Read the model definition and answer for the solid it produces. Units are mm, in the model's axes. Coordinates: 2 decimals unless noted, no trailing zeros. Write each loop counter-clockwise with the first axis right and the second up, starting at its lowest first coordinate (ties: lowest second). Pieces come first, ordered by that corner, then holes.
Item 1: Section B-B (z = 30) is taken. Give the vertices of the cut face in (x, y), then the cut area to 3 significant figures.
Item 2: Determine the mould class of faces 1 (the face through (1, 322.58, 9)), 2 (the face through (-25.97, 159.03, -33.86)), 3 (the face through (14, 159, 0)) for opening direction X: released by +X, released by -X, zero draft, split by the parting line, or undercut.
Item 3: Straight lines are drawn through the part: probe 1 along Z at (x, y) = (12, 136); probe 2 along Z at (x, y) = (-5, 158.5); probe 3 along X at (y, z) = (225, -16.5). For each, find the intervals that lie inside material, in ascending order.
Item 4: Section C-C (x = -25) is taken. Give the vertices of the cut face in (y, z).
Item 5: Each of these flat-tipped pins is pushed along its axis until it touches: P1, Ø12.5, axis at y = 134, z = 13.5, coming from the -X side; P2, Ø5, axis at y = 138.5, z = 31, coming from the +X side; P3, Ø17.5, axis at x = -13, y = 170, coming from the +Z side. Where does it stop, or does it pass through?
from build123d import *

# Parameters (mm, degrees)
SKETCH1_R           = 42.672
BOSS_EXTRUDE1_DEPTH = 322.58


with BuildPart() as part:
    # Sketch1 → Boss-Extrude1 (new body)
    with BuildSketch(Plane(origin=(0, 0, 0), x_dir=(1, 0, 0), z_dir=(0, 1, 0))):
        with Locations(Location((0, 0, 0), (0, 0, 270))):
            Circle(SKETCH1_R)
        with BuildLine():
            Line((0, 6.35), (0, 22.225))
            ThreePointArc((0, 22.225), (5.752253277, 21.467701489), (11.1125, 19.247414599))
            Line((11.1125, 19.247414599), (3.175, 5.499261314))
            ThreePointArc((3.175, 5.499261314), (4.490128061, 4.490128061), (5.499261314, 3.175))
            Line((5.499261314, 3.175), (19.247414599, 11.1125))
            ThreePointArc((19.247414599, 11.1125), (21.467701489, 5.752253277), (22.225, 0))
            Line((22.225, 0), (6.35, 0))
            ThreePointArc((6.35, 0), (6.133628997, -1.643500936), (5.499261314, -3.175))
            Line((5.499261314, -3.175), (19.247414599, -11.1125))
            ThreePointArc((19.247414599, -11.1125), (15.715448212, -15.715448212), (11.1125, -19.247414599))
            Line((11.1125, -19.247414599), (3.175, -5.499261314))
            ThreePointArc((3.175, -5.499261314), (1.643500936, -6.133628997), (0, -6.35))
            Line((0, -6.35), (0, -22.225))
            ThreePointArc((0, -22.225), (-5.752253277, -21.467701489), (-11.1125, -19.247414599))
            Line((-11.1125, -19.247414599), (-3.175, -5.499261314))
            ThreePointArc((-3.175, -5.499261314), (-4.490128061, -4.490128061), (-5.499261314, -3.175))
            Line((-5.499261314, -3.175), (-19.247414599, -11.1125))
            ThreePointArc((-19.247414599, -11.1125), (-21.467701489, -5.752253277), (-22.225, 0))
            Line((-22.225, 0), (-6.35, 0))
            ThreePointArc((-6.35, 0), (-6.133628997, 1.643500936), (-5.499261314, 3.175))
            Line((-5.499261314, 3.175), (-19.247414599, 11.1125))
            ThreePointArc((-19.247414599, 11.1125), (-15.715448212, 15.715448212), (-11.1125, 19.247414599))
            Line((-11.1125, 19.247414599), (-3.175, 5.499261314))
            ThreePointArc((-3.175, 5.499261314), (-1.643500936, 6.133628997), (0, 6.35))
        make_face(mode=Mode.SUBTRACT)
    extrude(amount=BOSS_EXTRUDE1_DEPTH)


solid = part.part
Established:
1. outline: (-30.35, 0) - (30.35, 0) - (30.35, 322.58) - (-30.35, 322.58) - close
1. area: 19,600 mm2
2. face 1: zero draft
2. face 2: split by the parting line
2. face 3: undercut
3. probe 1: z = -40.95 to -6.93, 0 to 6.93, 18.71 to 40.95
3. probe 2: z = -42.38 to -8.66, 3.91 to 8.66, 21.66 to 42.38
3. probe 3: x = -39.35 to -14.89, -9.53 to 0, 9.53 to 39.35
4. outline: (0, -34.58) - (322.58, -34.58) - (322.58, 34.58) - (0, 34.58) - close
5. P1: stops at x = -42.05
5. P2: stops at x = 31.76
5. P3: stops at z = 42.46
